Verification items for the finished model (mm, model axes). Give positions to 0.01 mm unless a question says otherwise; leave off trailing zeros. Loops run counter-clockwise (first coordinate to the right, second up) from the corner with the lowest first, then second, coordinate; pieces in that order, holes last. Notation, with made-up numbers: M 32,-18 L 89,-18 A17 ccw 89,1 Z; hole C 8,31 d9. An arc over 180 degrees is marked long. Use CSV: the item, a comma, the result in double quotes.
from build123d import *

# Parameters (mm, degrees)
PAD_DEPTH    = 4
FILLET_R     = 1
FILLET001_R  = 1
CHAMFER_SIZE = 1


with BuildPart() as part:
    # Sketch → Pad (new body)
    with BuildSketch(Plane.XY):
        with BuildLine():
            Line((-5, 10), (5, 10))
            Line((5, 10), (5, 8.174655))
            ThreePointArc((5, 0.170411), (8.719489, 4.172533), (5, 8.174655))
            Line((5, 0.170411), (5, -10))
            Line((5, -10), (-5, -10))
            Line((-5, -10), (-5, 10))
        make_face()
    extrude(amount=PAD_DEPTH)

    # Fillet
    fillet_edges = [part.edges().sort_by_distance(p)[0] for p in [
        (8.719489, 4.172533, 4),
    ]]
    fillet(fillet_edges, radius=FILLET_R)

    # Fillet001
    fillet001_edges = [part.edges().sort_by_distance(p)[0] for p in [
        (0, -10, 4),
    ]]
    fillet(fillet001_edges, radius=FILLET001_R)

    # Chamfer
    chamfer_edges = [part.edges().sort_by_distance(p)[0] for p in [
        (-5, 0.5, 4),
    ]]
    chamfer(chamfer_edges, length=CHAMFER_SIZE)


solid = part.part
(1) Scan lines: L1, parallel to X at y = -0.5, z = 2.5; L2, parallel to Y at x = 5.25, z = 3.6; L3, parallel to Y at x = 8, z = 0.65. Record each from-to range of solid material in increasing order. Write a range as from..to.
Calculated:
L1,"x = -5..5"
L2,"y = 0.4..7.95"
L3,"y = 1.88..6.47"
(2) Depth check by flat-ended pin: pin 1 Ø2 at (y, z) = (-5.5, 2) entering from +X. Enter the tip coordinate at first touch or a pass-through.
Calculated:
pin 1,"stops at x = 5"
(3) Section check B-B on y = -2.25. Record the cut outline in (x, z).
Calculated:
outline,"M -5,0 L 5,0 L 5,4 L -4,4 L -5,3 Z"
(4) Section check A-A on z = 0.8. Record the cut outline in (x, y), plus the area to 3 significant figures.
Calculated:
outline,"M -5,-9 L -4,-10 L 5,-10 L 5,0.17 A4.01 ccw 5,8.17 L 5,10 L -5,10 Z"
area,"222 mm²"
